Could you check a few things on this model? Use its own coordinates, in mm. A direction names the side the tool comes from. Give positions to 0.01 mm unless a question says otherwise; leave off trailing zeros. Write each loop counter-clockwise with the first axis right and the second up, starting at its lowest first coordinate (ties: lowest second). Pieces come first, ordered by that corner, then holes. Notation, with made-up numbers: (23, -1) -> (32, -1) arc R20 ccw to (32, 17) -> close; hole circle Ø3 at (-14, 47). An arc over 180 degrees is marked (long way). One line per question, with ' | ' between items.
Autodesk Inventor part; units mm, degrees
ref_plane "YZ Plane" through (0, 0, 0) normal (1, 0, 0) x (0, 1, 0)
ref_plane "XZ Plane" through (0, 0, 0) normal (0, 1, 0) x (-1, 0, 0)
ref_plane "XY Plane" through (0, 0, 0) normal (0, 0, 1) x (1, 0, 0)
sketch "Sketch1" plane through (0, 0, 0) normal (0, 1, 0) x (-1, 0, 0)
  line L0 (-101.6, 165.1) -> (101.6, 165.1)
  line L1 (117.475, 149.225) -> (117.475, -149.225)
  line L2 (101.6, -165.1) -> (-101.6, -165.1)
  line L3 (-117.475, -149.225) -> (-117.475, 149.225)
  line L4 (-117.475, 165.1) -> (117.475, -165.1) construction
  line L5 (117.475, 165.1) -> (-117.475, -165.1) construction
  arc A0 (-101.6, 165.1) -> (-117.475, 149.225) centre (-101.6, 149.225) ccw
  arc A1 (-117.475, -149.225) -> (-101.6, -165.1) centre (-101.6, -149.225) ccw
  arc A2 (101.6, -165.1) -> (117.475, -149.225) centre (101.6, -149.225) ccw
  arc A3 (117.475, 149.225) -> (101.6, 165.1) centre (101.6, 149.225) ccw
  point P0 (0, 0)
  point P1 (0, 0)
  dimension "d0" = 330.2
  dimension "d1" = 234.95
  dimension "d2" = 15.875
extrude "Extrusion1" add sketch "Sketch1" along normal blind 7.6835
fillet "Fillet1" radius 12.7 8 edges at (117.475, 7.6835, 0) (112.8253, 7.6835, -160.4503) (0, 7.6835, -165.1) (-112.8253, 7.6835, -160.4503) (-117.475, 7.6835, 0) (-112.8253, 7.6835, 160.4503) (0, 7.6835, 165.1) (112.8253, 7.6835, 160.4503)
sketch "Sketch2" plane through (0, 0, 0) normal (0, -1, 0) x (1, 0, 0)
  line L0 (101.6103, 150.8125) -> (101.6103, -150.8125)
  arc A0 (101.6103, 150.8125) -> (101.6, 150.8228) centre (101.6, 150.8125) ccw
  line L1 (-101.6, 150.8228) -> (101.6, 150.8228)
  arc A1 (-101.6, 150.8228) -> (-101.6103, 150.8125) centre (-101.6, 150.8125) ccw
  line L2 (-101.6103, -150.8125) -> (-101.6103, 150.8125)
  arc A2 (-101.6103, -150.8125) -> (-101.6, -150.8228) centre (-101.6, -150.8125) ccw
  line L3 (101.6, -150.8228) -> (-101.6, -150.8228)
  arc A3 (101.6, -150.8228) -> (101.6103, -150.8125) centre (101.6, -150.8125) ccw
  line L4 (103.505, -134.9375) -> (117.475, -134.9375)
  line L5 (117.475, -134.9375) -> (117.475, -150.8125)
  arc A4 (101.6, -166.6875) -> (117.475, -150.8125) centre (101.6, -150.8125) ccw
  line L6 (101.6, -166.6875) -> (-101.6, -166.6875)
  arc A5 (-117.475, -150.8125) -> (-101.6, -166.6875) centre (-101.6, -150.8125) ccw
  line L7 (-117.475, -150.8125) -> (-117.475, 150.8125)
  arc A6 (-101.6, 166.6875) -> (-117.475, 150.8125) centre (-101.6, 150.8125) ccw
  line L8 (-101.6, 166.6875) -> (101.6, 166.6875)
  arc A7 (117.475, 150.8125) -> (101.6, 166.6875) centre (101.6, 150.8125) ccw
  line L9 (117.475, 150.8125) -> (117.475, 134.9375)
  line L10 (117.475, 134.9375) -> (103.505, 134.9375)
  line L11 (103.505, 134.9375) -> (103.505, -134.9375)
  circle A8 centre (76.6206, 156.377) radius 5.1319
  line L12 (-38.4175, -52.3875) -> (-38.4175, 52.3875)
  line L13 (-38.4175, 52.3875) -> (-104.4575, 52.3875)
  line L14 (-104.4575, 52.3875) -> (-104.4575, -52.3875)
  line L15 (-104.4575, -52.3875) -> (-38.4175, -52.3875)
  line L16 (88.265, -146.05) -> (88.265, 146.05)
  line L17 (88.265, 146.05) -> (-28.8925, 146.05)
  line L18 (-28.8925, 146.05) -> (-28.8925, -146.05)
  line L19 (-28.8925, -146.05) -> (88.265, -146.05)
  line L20 (104.922, 134.9375) -> (117.475, 134.9375)
  line L21 (117.475, 134.9375) -> (117.475, -134.9375)
  line L22 (117.475, -134.9375) -> (104.922, -134.9375)
  line L23 (104.922, -134.9375) -> (104.922, 134.9375)
  point P0 (0, 0)
extrude "Extrusion2" add sketch "Sketch2" along normal blind 12.7 contours L23 L10 L21 L4
sketch "Sketch4" plane through (0, 0, 0) normal (0, 0, 1) x (1, 0, 0)
  circle A0 centre (109.8636, -6.6929) radius 3.8393
  circle A1 centre (109.8636, -6.6929) radius 3.8393
  point P0 (0, 0)
extrude "Extrusion3" add sketch "Sketch4" along normal mid plane 300
fillet "Fillet2" radius 12.7 1 edges at (117.475, -12.7, 0)
fillet "Fillet3" radius 3.175 1 edges at (104.922, -12.6991, 0)
sketch "Sketch5" plane through (0, 0, 0) normal (0, -1, 0) x (1, 0, 0)
  line L0 (104.922, 134.9375) -> (117.475, 134.9375)
  line L1 (117.475, 149.225) -> (117.475, 134.9375)
  arc A0 (117.475, 149.225) -> (101.6, 165.1) centre (101.6, 149.225) ccw
  line L2 (-101.6, 165.1) -> (101.6, 165.1)
  arc A1 (-101.6, 165.1) -> (-117.475, 149.225) centre (-101.6, 149.225) ccw
  line L3 (-117.475, -149.225) -> (-117.475, 149.225)
  arc A2 (-117.475, -149.225) -> (-101.6, -165.1) centre (-101.6, -149.225) ccw
  line L4 (101.6, -165.1) -> (-101.6, -165.1)
  arc A3 (101.6, -165.1) -> (117.475, -149.225) centre (101.6, -149.225) ccw
  line L5 (117.475, -134.9375) -> (117.475, -149.225)
  line L6 (117.475, -134.9375) -> (104.922, -134.9375)
  line L7 (104.922, -134.9375) -> (104.922, 134.9375)
  line L8 (89.535, -147.32) -> (-92.075, -147.32)
  line L9 (-92.075, -147.32) -> (-92.075, 147.32)
  line L10 (-92.075, 147.32) -> (89.535, 147.32)
  line L11 (89.535, 147.32) -> (89.535, -147.32)
  line L12 (89.535, -147.32) -> (-92.075, 147.32) construction
  line L13 (-92.075, -147.32) -> (89.535, 147.32) construction
  circle A4 centre (-103.4539, 0) radius 1.8839
  point P0 (0, 0)
  point P1 (-1.27, 0)
  dimension "d12" = 17.78
  dimension "d13" = 17.78
  dimension "d14" = 25.4
  dimension "d15" = 27.94
extrude "Extrusion4" cut sketch "Sketch5" against normal blind 0.254 contours L8 L9 L10 L11 | A4
properties part number "dellLatitudeScreen"
Q1. Will these pins go through, and if not, where does the flat tip stop? pin 1 (4 mm diameter, centred on y = -4, z = -54, fed in from -X); pin 2 (2.5 mm diameter, centred on x = 108.5, y = -5.5, fed in from -Z); pin 3 (1.1 mm diameter, centred on x = -104, z = 0, fed in from -Y).
Answer below:
pin 1: stops at x = 104.92 | pin 2: stops at z = -150 | pin 3: stops at y = 0.25
Q2. If we mould it in two halves opening along Y, with no side actions, what happens to faces 6 (the cylindrical face through (1.422, 5.647, 160.331)), 7 (the cylindrical face through (113.4, -5.2, 142.4)), 8 (the flat face through (113, -3, -134.938)), 9 (the cylindrical face through (115.14, -7.34, 1.89))? For each: +Y half, -Y half, draft (parallel to the pull), parting line (faces both ways), or undercut.
Answer below:
face 6: +Y half | face 7: undercut | face 8: undercut | face 9: -Y half
Q3. If I drill on line 1 along Y through (x, z) = (-104, 70.5); line 2 along Y through (x, z) = (21, 113); line 3 along X through (y, z) = (-9, -148.5), over which ranges is the centre line in solid material (lowest first)?
Answer below:
line 1: y = 0 to 7.68 | line 2: y = 0.25 to 7.68 | line 3: x = 106.79 to 112.93
Q4. Imagine slicing it at A-A on x = 35. Please give me the cut outline in (y, z).
Answer below:
outline: (0, -165.1) arc R12.7 ccw to (7.68, -153.43) -> (7.68, 153.43) arc R12.7 ccw to (0, 165.1) -> (0, 147.32) -> (0.25, 147.32) -> (0.25, -147.32) -> (0, -147.32) -> close
Q5. On a 3-axis mill with a long thin cutter (end or side, diameter ignored), from which of +Z, -Z, +X, -X, +Y, -Y can I reach the whole of each face in a straight line? I mean faces 1 (the flat face through (104.922, -4, -2)), 2 (the flat face through (-3, 0.254, 2)), 3 (the flat face through (110, -7, 150)), 4 (the flat face through (110, -7, -150)), 5 (the flat face through (113, -3, 134.938)). Say none if no direction works.
Answer below:
face 1: +Z, -Z, -X, -Y | face 2: -Y | face 3: +Z, +X, -X, -Y | face 4: -Z, +X, -X, -Y | face 5: +Z
